Here's how the part is built. I have some questions about the finished solid (model axes, mm). A direction names the side the tool comes from. Give positions to 0.01 mm unless a question says otherwise; leave off trailing zeros. Write each loop counter-clockwise with the first axis right and the second up, starting at its lowest first coordinate (ties: lowest second). Pieces come first, ordered by that corner, then holes. Notation, with made-up numbers: (80, -15.75) - (94, -15.75) arc R21 ccw to (94, 8.25) - close; hole circle Ø8 at (9.5, 19.25). An arc over 180 degrees is marked (long way). One line per item, written item: value. Start each with the question number.
1) I'm going to push flat-ended pins straight in: P1, Ø13, axis at y = 0, z = 0, coming from the +X side; P2, Ø9.5, axis at y = 15.56, z = -47.88, coming from the +X side; P3, Ø5, axis at x = -14, z = 0, coming from the -Y side; P4, Ø1.5, axis at x = -18.5, y = 9.5, coming from the -Z side. Where does each tip first touch, or does it pass through?
2) Imagine slicing it at D-D on y = -33. Write out the boundary of the cut face in (x, z), plus the area to 3 significant figures.
3) Please list where these lines run through material, in increasing order: L1, parallel to Y at x = -25, z = 0; L2, parallel to X at y = 2.5, z = -54.5; L3, parallel to Z at x = -22, y = 5. Write a range as [from, to].
4) Imagine slicing it at C-C on x = -21.5. Write out the boundary of the cut face in (y, z), plus the area to 3 significant figures.
5) We'd pull the mould along Y, two halves only. Please class faces 4 (the cylindrical face through (-2.465, 2.652, 60.267)), 5 (the flat face through (-35, -8, -8)), 6 (the cylindrical face through (-2.465, 46.376, 0.881)), 7 (the flat face through (-18, 10, -3)): +Y half, -Y half, draft (parallel to the pull), parting line (faces both ways), or undercut.
6) Imagine slicing it at A-A on z = 0. Write out the boundary of the cut face in (x, y) (3 decimals), plus the area to 3 significant figures.
7) Imagine slicing it at B-B on y = 0. Write out the boundary of the cut face in (x, z) (3 decimals).
8) On a 3-axis mill with a long thin cutter (end or side, diameter ignored), from which of +Z, -Z, +X, -X, +Y, -Y can I reach the whole of each face in a straight line? I mean faces 1 (the cylindrical face through (-34, -11, 0)), 2 (the flat face through (0, 1, -13)), 3 (the flat face through (-18, 11.006, 0)). Say none if no direction works.
from build123d import *

# Parameters (mm, degrees)
SKETCH1_R                           = 60.325
BOSS_EXTRUDE1_DEPTH                 = 5
SKETCH2_R                           = 4.064
CUT_EXTRUDE1_DEPTH                  = 86.458827806
SKETCH11_R                          = 17.5
BOSS_EXTRUDE3_DEPTH                 = 30
CUT_EXTRUDE5_DEPTH                  = 93.212858377
SKETCH13_R                          = 11
CUT_MOTORSHOULDERRECESS_D22X3_DEPTH = 3


with BuildPart() as part:
    # Sketch1 → Boss-Extrude1 (new body)
    with BuildSketch(Plane(origin=(0, 0, 0), x_dir=(0, 0, -1), z_dir=(1, 0, 0))):
        Circle(SKETCH1_R)
    extrude(amount=-BOSS_EXTRUDE1_DEPTH)

    # Sketch2 → Cut-Extrude1 (cut, through all)
    with BuildSketch(Plane(origin=(0, 0, 0), x_dir=(0, 0, -1), z_dir=(1, 0, 0))):
        with Locations((0, 50.342959834)):
            Circle(SKETCH2_R)
        with Locations((47.879, 15.556830136)):
            Circle(SKETCH2_R)
        with Locations((29.590849347, -40.728310053)):
            Circle(SKETCH2_R)
        with Locations((-29.590849347, -40.728310053)):
            Circle(SKETCH2_R)
        with Locations((-47.879, 15.556830136)):
            Circle(SKETCH2_R)
    extrude(amount=-CUT_EXTRUDE1_DEPTH, mode=Mode.SUBTRACT)

    # Sketch11 → Boss-Extrude3 (add)
    with BuildSketch(Plane.ZY.offset(5)):
        with Locations(Location((0, 0, 0), (0, 0, 180))):
            Circle(SKETCH11_R)
    extrude(amount=BOSS_EXTRUDE3_DEPTH)

    # Sketch12 → Cut-Extrude5 (cut, through all)
    with BuildSketch(Plane.ZY.offset(35)):
        with BuildLine():
            Line((0, 11.006403687), (-3, 11.006403687))
            Line((-3, 11.006403687), (-3, 8.006403687))
            ThreePointArc((-3, 8.006403687), (0, -8.55), (3, 8.006403687))
            Line((3, 8.006403687), (3, 11.006403687))
            Line((3, 11.006403687), (0, 11.006403687))
        make_face()
    extrude(amount=-CUT_EXTRUDE5_DEPTH, mode=Mode.SUBTRACT)

    # Sketch13 → Cut_MotorShoulderRecess_D22x3 (cut)
    with BuildSketch(Plane(origin=(-35, 0, 0), x_dir=(0, 0, -1), z_dir=(1, 0, 0))):
        Circle(SKETCH13_R)
    extrude(amount=CUT_MOTORSHOULDERRECESS_D22X3_DEPTH, mode=Mode.SUBTRACT)


solid = part.part
Numbers:
1. P1: through
1. P2: x = 0
1. P3: y = -17.5
1. P4: z = -15.16
2. outline: (-5, -50.5) - (0, -50.5) - (0, 50.5) - (-5, 50.5) - close
2. area: 505 mm^2
3. L1: [-17.5, -8.55], [11.01, 17.5]
3. L2: [-5, 0]
3. L3: [-16.77, -6.94], [6.94, 16.77]
4. outline: circle Ø35 at (0, 0); hole (8.01, -3) - (11.01, -3) - (11.01, 3) - (8.01, 3) arc R8.55 ccw (long way) to start
4. area: 717 mm^2
5. face 4: parting line
5. face 5: draft
5. face 6: undercut
5. face 7: undercut
6. outline: (-35, -17.5) - (-5, -17.5) - (-5, -60.325) - (0, -60.325) - (0, -8.55) - (-32, -8.55) - (-32, -11) - (-35, -11) - close; (-35, 11.006) - (0, 11.006) - (0, 46.279) - (-5, 46.279) - (-5, 17.5) - (-35, 17.5) - close; (-5, 54.407) - (0, 54.407) - (0, 60.325) - (-5, 60.325) - close
6. area: 921 mm^2
7. outline: (-35, -17.5) - (-5, -17.5) - (-5, -60.325) - (0, -60.325) - (0, -8.55) - (-32, -8.55) - (-32, -11) - (-35, -11) - close; (-35, 11) - (-32, 11) - (-32, 8.55) - (0, 8.55) - (0, 60.325) - (-5, 60.325) - (-5, 17.5) - (-35, 17.5) - close
8. face 1: -X
8. face 2: +Z, -Z, +X, +Y, -Y
8. face 3: +X, -X
